Part model, mm, in its own coordinate system. Round coordinates to 2 decimals unless told otherwise and drop trailing zeros. Write each loop counter-clockwise with the first axis right and the second up, starting at its lowest first coordinate (ties: lowest second). Pieces come first, ordered by that corner, then holes. Notation, with made-up numbers: M -18.5,84.5 L 40.5,84.5 A18 ccw 40.5,106.5 Z; hole C 13.5,-39.5 d2. An arc over 180 degrees is marked long. Answer as a JSON object with one key per item and string values. Group by question number.
1. Drill centre lines: line 1 (Y direction, x = 0, z = 17.55) (3 decimals); line 2 (Y direction, x = 0.25, z = 16.5); line 3 (Y direction, x = 4.25, z = -14). Where is each one in solid material? Low to high. Write a range as from..to.
2. Band-saw the part on C-C, the plane y = 1.5. Write the cut outline in (x, z), plus the area to 3 significant figures.
3. Band-saw the part on D-D, the plane x = -2. Write the cut outline in (y, z), plus the area to 3 significant figures.
4. Drop flat-ended pins along their axis: pin 1 (6 mm diameter, centred on x = -2.5, z = -12, fed in from +Y); pin 2 (1.8 mm diameter, centred on x = 0, y = -3.175, fed in from -Z); pin 3 (4 mm diameter, centred on y = -4, z = -15, fed in from +X). Give the stop position or say it passes through.
5. Band-saw the part on B-B, the plane z = 8. Write the cut outline in (x, y), plus the area to 3 significant figures.
6. Band-saw the part on A-A, the plane x = 0. Write the cut outline in (y, z) (3 decimals).
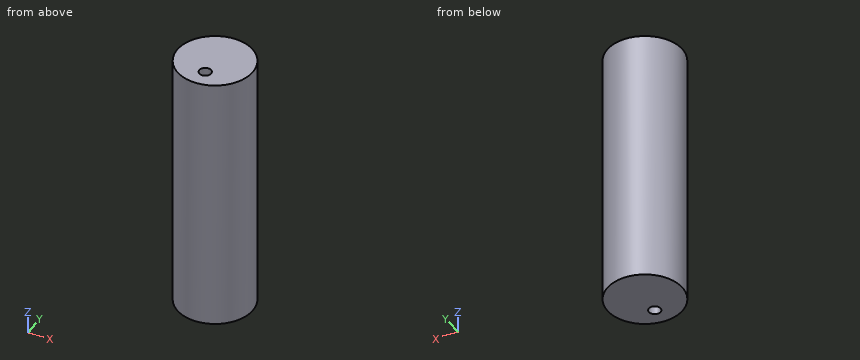
Autodesk Inventor part; units mm, degrees
ref_plane "YZ Plane" through (0, 0, 0) normal (1, 0, 0) x (0, 1, 0)
ref_plane "XZ Plane" through (0, 0, 0) normal (0, 1, 0) x (-1, 0, 0)
ref_plane "XY Plane" through (0, 0, 0) normal (0, 0, 1) x (1, 0, 0)
sketch "Sketch1" plane through (0, 0, 0) normal (0, 0, 1) x (1, 0, 0)
  circle A0 centre (0, 0) radius 6.35
  dimension "d2" = 12.7
extrude "Extrusion1" add sketch "Sketch1" along normal mid plane 44
sketch "Sketch2" plane through (0, 0, 22) normal (0, 0, 1) x (1, 0, 0)
  circle A0 centre (0, -3.175) radius 1
  point P0 (0, 0)
  dimension "d3" = 2
  dimension "d4" = 3.175
hole "Hole1" at (0, -3.175, 22) direction (0, 0, -1) diameter 2 depth 6
mirror "Mirror1" about plane through (0, 0, 0) normal (0, 0, 1) of "Hole1"
thread "Thread1"
thread "Thread2"
properties part number "Tubo Soporte para Corte"
Worked answers:
{
 "1": {"line 1": "y = -6.35..-4.175, -2.175..6.35", "line 2": "y = -6.35..-4.14, -2.21..6.35", "line 3": "y = -4.72..4.72"},
 "2": {"outline": "M -6.17,-22 L 6.17,-22 L 6.17,22 L -6.17,22 Z", "area": "543 mm^2"},
 "3": {"outline": "M -6.03,-22 L 6.03,-22 L 6.03,22 L -6.03,22 Z", "area": "530 mm^2"},
 "4": {"pin 1": "stops at y = 6.35", "pin 2": "stops at z = -16", "pin 3": "stops at x = 6.03"},
 "5": {"outline": "C 0,0 d12.7", "area": "127 mm^2"},
 "6": {"outline": "M -6.35,-22 L -4.175,-22 L -4.175,-16 L -2.175,-16 L -2.175,-22 L 6.35,-22 L 6.35,22 L -2.175,22 L -2.175,16 L -4.175,16 L -4.175,22 L -6.35,22 Z"}
}
